```python
from build123d import *

# Parameters (mm, degrees)
SKETCH1_R               = 36
BOSS_EXTRUDE1_DEPTH     = 18
SKETCH2_W               = 36
SKETCH2_H               = 36
BOSS_EXTRUDE2_DEPTH     = 109
SKETCH3_R               = 15
BOSS_EXTRUDE3_DEPTH     = 20
CUT_EXTRUDE1_DEPTH      = 40
CIRPATTERN1_COUNT       = 4
SKETCH5_R               = 30
BOSS_EXTRUDE4_DEPTH     = 40
CUT_EXTRUDE2_DEPTH      = 139.351002938
CUT_EXTRUDE2_DEPTH_BACK = 139.351002938
HOLE1_D                 = 30


with BuildPart() as part:
    # Sketch1 → Boss-Extrude1 (new, symmetric)
    with BuildSketch(Plane(origin=(0, 0, 0), x_dir=(0, 0, -1), z_dir=(1, 0, 0))):
        Circle(SKETCH1_R)
    extrude(amount=BOSS_EXTRUDE1_DEPTH, both=True)

    # Sketch2 → Boss-Extrude2 (add)
    with BuildSketch(Plane.XY):
        Rectangle(SKETCH2_W, SKETCH2_H)
    extrude(amount=BOSS_EXTRUDE2_DEPTH)

    # Sketch3 → Boss-Extrude3 (add)
    with BuildSketch(Plane.XY.offset(109)):
        Circle(SKETCH3_R)
    extrude(amount=BOSS_EXTRUDE3_DEPTH)

    # Sketch4 → Cut-Extrude1 (cut)
    with BuildSketch(Plane.XY.offset(109)):
        with BuildLine():
            Line((13, 18), (18, 18))
            Line((18, 18), (18, 13))
            ThreePointArc((18, 13), (14.464466094, 14.464466094), (13, 18))
        make_face()
    cut_extrude1 = extrude(amount=-CUT_EXTRUDE1_DEPTH, mode=Mode.SUBTRACT)

    # CirPattern1: Cut-Extrude1 ×4 about axis
    cirpattern1_axis = Axis((0, 0, 0), (0, 0, 1))
    for i in range(1, CIRPATTERN1_COUNT):
        add(cut_extrude1.rotate(cirpattern1_axis, i * 360 / CIRPATTERN1_COUNT), mode=Mode.SUBTRACT)

    # Sketch5 → Boss-Extrude4 (add, symmetric)
    with BuildSketch(Plane(origin=(0, 0, 0), x_dir=(1, 0, 0), z_dir=(0, 1, 0))):
        with Locations(Location((0, 18, 0), (0, 0, 270))):
            Circle(SKETCH5_R)
    extrude(amount=BOSS_EXTRUDE4_DEPTH, both=True)

    # Sketch6 → Cut-Extrude2 (cut, two sides: drawn at the far end of the back side and taken through both)
    with BuildSketch(Plane(origin=(0, 0, 0), x_dir=(0, 0, -1), z_dir=(1, 0, 0)).offset(-CUT_EXTRUDE2_DEPTH_BACK)):
        with BuildLine():
            Line((-6, 18), (48, 18))
            Line((48, 18), (48, -18))
            Line((48, -18), (-6, -18))
            ThreePointArc((-6, -18), (-24, 0), (-6, 18))
        make_face()
    extrude(amount=CUT_EXTRUDE2_DEPTH + CUT_EXTRUDE2_DEPTH_BACK, mode=Mode.SUBTRACT)

    # Hole1 (through all)
    with Locations(Plane(origin=(0, 40, 0), x_dir=(1, 0, 0), z_dir=(0, 1, 0))):
        with Locations((0, 18)):
            Hole(HOLE1_D / 2)


solid = part.part
```
Geometry check sheet. Reference: the model listing, model coordinates, mm. A direction names the side the tool comes from. Coordinates: 2 decimals unless noted, no trailing zeros. Write each loop counter-clockwise with the first axis right and the second up, starting at its lowest first coordinate (ties: lowest second). Pieces come first, ordered by that corner, then holes. Notation, with made-up numbers: M 26.5,77 L 79.5,77 A35 ccw 79.5,112 Z; hole C 57.5,-34.5 d4. An arc over 180 degrees is marked long. Use one line per item in the form item = value. Start each with the question number.
1) Section check B-B on y = 0. Enter the section's corners in (x, z).
2) Section check A-A on z = -18. Enter the section's corners in (x, y).
3) Thickness scan on probe 1 along Y at (x, z) = (-26.5, -6); probe 2 along Z at (x, y) = (0, 23.25); probe 3 along Y at (x, z) = (8, 66). Record the ranges inside material, lowest first. Write a range as from..to.
4) Release check for a two-part mould opening along Z. For faces 5 (the flat face through (16, -16, 69)), 6 (the flat face through (-0.4, -18, -33.4)), 7 (the cylindrical face through (3.252, -29.154, -3.357)) record: pulls with the +Z half, pulls with the -Z half, needs draft (parallel to the pull), parting line crosses it, or undercut.
5) Set-up check for faces 1 (the flat face through (-16, -16, 69)), 2 (the flat face through (0, 18, 70)), 3 (the flat face through (18, 0, 47)), 4 (the cylindrical face through (14, -15, 89)): record each of +Z, -Z, +X, -X, +Y, -Y from which the full face is reachable in a straight line by a thin tool's end or side.
6) Go/stop test with flat-tipped pins: pin 1 Ø4 at (x, y) = (15, 15.5) entering from +Z; pin 2 Ø16 at (x, z) = (4.5, -11.5) entering from +Y; pin 3 Ø6 at (x, z) = (11.5, 91.5) entering from +Y; pin 4 Ø6 at (x, y) = (6.5, -28) entering from +Z. Record where each tip stops, or that it passes through.
7) Section check D-D on z = 105. Enter the section's corners in (x, y), and give its area (3 significant figures).
8) Section check C-C on x = 0. Enter the section's corners in (y, z), and give its area (3 significant figures).
Responses:
q1.outline = M -18,24 L 18,24 L 18,109 L 15,109 L 15,129 L -15,129 L -15,109 L -18,109 Z
q2.outline = M -30,-40 L -15,-40 L -15,-18 L -30,-18 Z; M -30,18 L -15,18 L -15,40 L -30,40 Z; M 15,-40 L 30,-40 L 30,-18 L 15,-18 Z; M 15,18 L 30,18 L 30,40 L 15,40 Z
q3.probe_1 = -40..-18, 18..40
q3.probe_2 = -48..-33, -3..27.49
q3.probe_3 = -18..18
q4.face_5 = pulls with the +Z half
q4.face_6 = needs draft
q4.face_7 = undercut
q5.face_1 = +Z, -X, -Y
q5.face_2 = +Z, +X, -X, +Y
q5.face_3 = +Z, +X, +Y, -Y
q5.face_4 = +Z, +X, -Y
q6.pin_1 = 109
q6.pin_2 = 40
q6.pin_3 = 18
q6.pin_4 = 25.9
q7.outline = M -18,-13 A5 cw -13,-18 L 13,-18 A5 cw 18,-13 L 18,13 A5 cw 13,18 L -13,18 A5 cw -18,13 Z
q7.area = 1,220 mm2
q8.outline = M -40,-48 L -18,-48 L -18,-33 L -40,-33 Z; M -40,-3 L -18,-3 L -18,6 A18 cw 18,6 L 18,-3 L 40,-3 L 40,12 L 33.94,12 A36 ccw 18,31.18 L 18,109 L 15,109 L 15,129 L -15,129 L -15,109 L -18,109 L -18,31.18 A36 ccw -33.94,12 L -40,12 Z; M 18,-48 L 40,-48 L 40,-33 L 18,-33 Z
q8.area = 5,500 mm2
